Part model, mm, in its own coordinate system. A direction names the side the tool comes from. Round coordinates to 2 decimals unless told otherwise and drop trailing zeros. Order: outer loops, then holes, each group sorted by start corner. A loop starts at its lowest first (then second) coordinate and runs counter-clockwise, first axis right, second up. Notation, with made-up numbers: (-8.5, 63.5) - (14.5, 63.5) arc R35 cw to (14.5, 100.5) - close; hole circle Ø5 at (54, -38). An arc over 180 degrees is marked (long way). Return JSON: item names as keys, results as strings. Group by question number.
Item 1: Tool access for faces 1 (the face through (1, -1, 45.72)), 2 (the face through (2.54, -1, 24)), 3 (the face through (27, -1, 1.778)): list every direction of +Z, -Z, +X, -X, +Y, -Y with a clear straight run to the whole face (end or side of a thin tool).
Item 2: Saw through at A-A on y = -1.27. List the corners of the cut face in (x, z).
Item 3: Saw through at D-D on x = 4. List the corners of the cut face in (y, z), and give its area (3 significant figures).
Item 4: Saw through at B-B on x = 27.5. List the corners of the cut face in (y, z).
Item 5: Drop a flat-ended pin along its axis: pin 1 (1.5 mm diameter, centred on x = 26.5, y = -2, fed in from +Z). Give the stop position or say it passes through.
Item 6: Two-plate mould, pull along X, no slides. Class faces 4 (the face through (27.926, -1.537, 0.877)), 5 (the face through (15, -1, 0)), 6 (the face through (30.48, -1, 1)): released by +X, released by -X, zero draft, split by the parting line, or undercut.
Item 7: Saw through at C-C on z = 13. List the corners of the cut face in (x, y), and give its area (3 significant figures).
Item 8: Probe probe 1 along X at (y, z) = (-2.05, 36). List the from-to ranges inside material, lowest first.
```python
from build123d import *

# Parameters (mm, degrees)
F0_W     = 2.54
F0_H     = 2.54
F0_W_2   = 27.94
F0_H_2   = 43.18
F1_DEPTH = 2.54
F3_DEPTH = 1.778


with BuildPart() as f1:
    # F0 (on Front) → F1 (new body)
    with BuildSketch(Plane.XZ):
        with Locations((1.27, 1.27)):
            Rectangle(F0_W, F0_H)
        with Locations((16.51, 1.27)):
            Rectangle(F0_W_2, F0_H)
        with Locations((1.27, 24.13)):
            Rectangle(F0_W, F0_H_2)
    extrude(amount=F1_DEPTH)

    # F2 (on face) → F3 (cut)
    with BuildSketch(Plane(origin=(0, 0, 0), x_dir=(1, 0, 0), z_dir=(0, 0, -1))):
        with BuildLine():
            ThreePointArc((26.188626, 1.27), (27.077626, 0.381), (27.966626, 1.27))
            Line((27.966626, 1.27), (26.188626, 1.27))
        make_face()
        with BuildLine():
            Line((26.188626, 1.27), (27.966626, 1.27))
            ThreePointArc((27.966626, 1.27), (27.077626, 2.159), (26.188626, 1.27))
        make_face()
    extrude(amount=-F3_DEPTH, mode=Mode.SUBTRACT)


solid = f1.part
```
Filled in:
{
 "1": {"face 1": "+Z, +X, -X, +Y, -Y", "face 2": "+Z, +X, +Y, -Y", "face 3": "-Z"},
 "2": {"outline": "(0, 0) - (26.19, 0) - (26.19, 1.78) - (27.97, 1.78) - (27.97, 0) - (30.48, 0) - (30.48, 2.54) - (2.54, 2.54) - (2.54, 45.72) - (0, 45.72) - close"},
 "3": {"outline": "(-2.54, 0) - (0, 0) - (0, 2.54) - (-2.54, 2.54) - close", "area": "6.45 mm^2"},
 "4": {"outline": "(-2.54, 0) - (-2.05, 0) - (-2.05, 1.78) - (-0.49, 1.78) - (-0.49, 0) - (0, 0) - (0, 2.54) - (-2.54, 2.54) - close"},
 "5": {"pin 1": "stops at z = 2.54"},
 "6": {"face 4": "undercut", "face 5": "zero draft", "face 6": "released by +X"},
 "7": {"outline": "(0, -2.54) - (2.54, -2.54) - (2.54, 0) - (0, 0) - close", "area": "6.45 mm^2"},
 "8": {"probe 1": "x = 0 to 2.54"}
}
